Print and shaded views of the part. All mm, measured from the part's lowest x, y and z. Round coordinates to 2 decimals unless told otherwise and drop trailing zeros. Loops run counter-clockwise (first coordinate to the right, second up) from the corner with the lowest first, then second, coordinate; pieces in that order, holes last. Notation, with made-up numbers: (54.25, -30.75) - (110.25, -30.75) arc R23 ccw to (110.25, -12.75) - close; hole circle Ø6 at (11.25, 77). An arc over 180 degrees is marked (long way). Use one line per item in the form item = value.
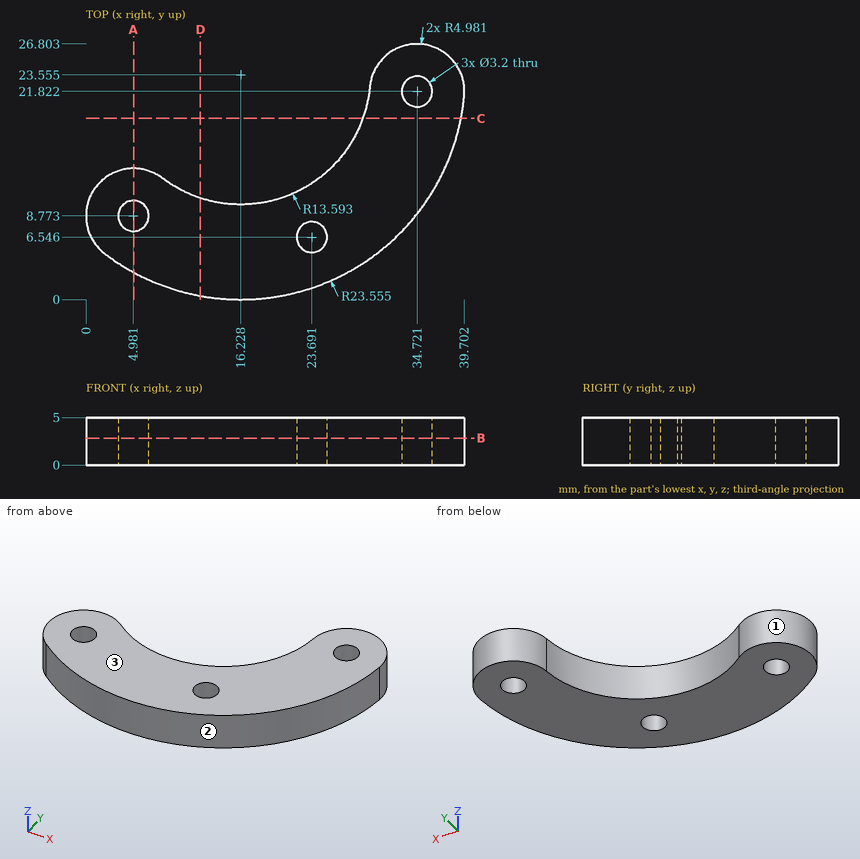
1. Cut at A-A, the plane x = 5. Give the cut face in (y, z).
Geometry check:
outline = (2.85, 0) - (7.17, 0) - (7.17, 5) - (2.85, 5) - close; (10.37, 0) - (13.75, 0) - (13.75, 5) - (10.37, 5) - close
2. Cut at C-C, the plane y = 19. Give the cut face in (x, z) (1 decimal).
Geometry check:
outline = (29, 0) - (39.3, 0) - (39.3, 5) - (29, 5) - close
3. Pull direction X, two halves, no side cores. Call the marked faces 1, 2 and 3: +X half, -X half, draft (parallel to the pull), parting line (faces both ways), or undercut.
Geometry check:
face_1 = undercut
face_2 = parting line
face_3 = draft
4. Wall check: probe 1 along X at (y, z) = (8, 3.9) (1 decimal); probe 2 along X at (y, z) = (12.25, 3.95) (1 decimal); probe 3 along X at (y, z) = (20.75, 2.3) (1 decimal). Give the ranges that are in metal, low to high.
Geometry check:
probe_1 = 0.1 to 3.6, 6.4 to 23, 24.4 to 33.9
probe_2 = 1.4 to 8.7, 23.8 to 36.9
probe_3 = 29.5 to 33.5, 35.9 to 39.6
5. Flat gauge pins, fed straight in: pin 1 (2.5 mm diameter, centred on x = 4.98, y = 8.77, fed in from +Z); pin 2 (3 mm diameter, centred on x = 17.5, z = 1.5, fed in from +Y). Where does each tip first touch, or does it go through?
Geometry check:
pin_1 = through
pin_2 = 10.25
6. Cut at B-B, the plane z = 2.85. Give the cut face in (x, y) (1 decimal).
Geometry check:
outline = (2, 4.8) arc R23.6 ccw to (39.7, 21.4) arc R5 ccw to (29.8, 22.3) arc R13.6 cw to (8, 12.7) arc R5 ccw to start; hole circle Ø3.2 at (5, 8.8); hole circle Ø3.2 at (23.7, 6.5); hole circle Ø3.2 at (34.7, 21.8)
7. Cut at D-D, the plane x = 12. Give the cut face in (y, z) (1 decimal).
Geometry check:
outline = (0.4, 0) - (10.6, 0) - (10.6, 5) - (0.4, 5) - close
